Here's how the part is built. I have some questions about the finished solid (model axes, mm). A direction names the side the tool comes from. Round coordinates to 2 decimals unless told otherwise and drop trailing zeros. Write each loop counter-clockwise with the first axis right and the second up, starting at its lowest first coordinate (ties: lowest second). Pieces come first, ordered by that corner, then holes. Notation, with made-up numbers: (-22.5, 58) -> (0.5, 58) arc R32 ccw to (0.5, 92) -> close; hole circle Ø11 at (79.5, -2.5). An arc over 180 degrees is marked (long way). Answer as CSV lines item,"result".
Autodesk Inventor part; units mm, degrees
ref_plane "dp1_XY" through (7.9502, 4.7307, 0) normal (0, 0, 1) x (1, 0, 0)
ref_plane "dp1_YZ" through (7.9502, 4.7307, 0) normal (1, 0, 0) x (0, 1, 0)
ref_plane "dp1_ZX" through (7.9502, 4.7307, 0) normal (0, 1, 0) x (0, 0, 1)
sketch "Sketch_2" plane through (0, 0, 0) normal (0, 0, 1) x (1, 0, 0)
  line L0 (7.9502, 0) -> (0, 0)
  line L1 (0, 0) -> (0, 4.1326)
  line L2 (0, 4.1326) -> (0.6299, 4.7625)
  line L3 (0.6299, 4.7625) -> (3.9106, 4.7625)
  line L4 (3.9106, 4.7625) -> (4.5411, 4.1336)
  arc A0 (4.5411, 4.1336) -> (5.0165, 3.937) centre (5.0165, 4.6101) ccw
  line L5 (5.0165, 3.937) -> (6.0071, 3.937)
  arc A1 (6.0071, 3.937) -> (6.6802, 4.6101) centre (6.0071, 4.6101) ccw
  line L6 (6.6802, 4.6101) -> (6.6802, 4.7307)
  line L7 (6.6802, 4.7307) -> (7.9502, 4.7307)
  line L8 (7.9502, 4.7307) -> (7.9502, 0)
  line L9 (7.9502, 0) -> (0, 0)
revolve "Revolution1" add sketch "Sketch_2" angle 360 about axis through (7.9502, 0, 0) along (1, 0, 0)
thread "Thread1"
sketch "Sketch_3" plane through (0, 0, 0) normal (0, 0, 1) x (1, 0, 0)
  line L0 (15.9004, 0) -> (7.9502, 0)
  line L1 (7.9502, 0) -> (7.9502, 6.1468)
  line L2 (7.9502, 6.1468) -> (11.1252, 6.1468)
  line L3 (11.1252, 6.1468) -> (11.1252, 5.1626)
  line L4 (11.1252, 5.1626) -> (11.6332, 5.1626)
  line L5 (11.6332, 5.1626) -> (12.1412, 5.6706)
  line L6 (12.1412, 5.6706) -> (15.3924, 5.6706)
  line L7 (15.3924, 5.6706) -> (15.9004, 5.1626)
  line L8 (15.9004, 5.1626) -> (15.9004, 0)
  line L9 (15.9004, 0) -> (7.9502, 0)
revolve "Revolution2" add sketch "Sketch_3" angle 360 about axis through (15.9004, 0, 0) along (1, 0, 0)
sketch "Sketch_4" plane through (0, 0, 0) normal (0, 0, 1) x (1, 0, 0)
  line L0 (17.4752, 0) -> (15.9004, 0)
  line L1 (15.9004, 0) -> (15.9004, 4.4069)
  line L2 (15.9004, 4.4069) -> (17.4752, 4.4069)
  line L3 (17.4752, 4.4069) -> (17.4752, 0)
  line L4 (17.4752, 0) -> (15.9004, 0)
revolve "Revolution3" add sketch "Sketch_4" angle 360 about axis through (17.4752, 0, 0) along (1, 0, 0)
sketch "Sketch4" plane through (0, 0, 0) normal (-1, 0, 0) x (0, 0, 1)
  point P0 (0, 0)
hole "Hole1" at (0, 0, 0) direction (1, 0, 0) diameter 4.8133 depth 17.4752 countersink diameter 5.8293 countersink angle 90
sketch "Sketch_47" plane through (0, 0, 0) normal (0, 0, 1) x (1, 0, 0)
  line L0 (11.6332, 0) -> (11.1252, 0)
  line L1 (11.1252, 5.6603) -> (11.1252, 4.9085)
  line L2 (11.1252, 4.9085) -> (11.6332, 4.9085)
  line L3 (11.6332, 4.9085) -> (11.6332, 5.1626)
  line L4 (11.6332, 5.1626) -> (11.3792, 5.1626)
  line L5 (11.3792, 5.1626) -> (11.2368, 5.305)
  arc A0 (11.2368, 5.4846) -> (11.2368, 5.305) centre (11.3266, 5.3948) ccw
  line L6 (11.2368, 5.4846) -> (11.8149, 6.0626)
  line L7 (11.8149, 6.0626) -> (11.8149, 6.1468)
  line L8 (11.8149, 6.1468) -> (11.6117, 6.1468)
  line L9 (11.6117, 6.1468) -> (11.1252, 5.6603)
revolve "Revolution4" add sketch "Sketch_47" angle 360 about axis through (11.6332, 0, 0) along (1, 0, 0)
ref_plane "dp1_XY" through (7.9502, 4.7307, 0) normal (0, 0, 1) x (1, 0, 0)
ref_plane "dp1_YZ" through (7.9502, 4.7307, 0) normal (1, 0, 0) x (0, 1, 0)
ref_plane "dp1_ZX" through (7.9502, 4.7307, 0) normal (0, 1, 0) x (0, 0, 1)
ref_plane "dp2_XY" through (7.9502, -4.7307, 0) normal (0, 0, 1) x (1, 0, 0)
ref_plane "dp2_YZ" through (7.9502, -4.7307, 0) normal (1, 0, 0) x (0, 1, 0)
ref_plane "dp2_ZX" through (7.9502, -4.7307, 0) normal (0, 1, 0) x (0, 0, 1)
ref_plane "hh_XY" through (0, 4.7625, 0) normal (0, 0, 1) x (1, 0, 0)
ref_plane "hh_YZ" through (0, 4.7625, 0) normal (1, 0, 0) x (0, 1, 0)
ref_plane "hh_ZX" through (0, 4.7625, 0) normal (0, 1, 0) x (0, 0, 1)
ref_plane "rod_guide_XY" through (0, 0, 0) normal (1, 0, 0) x (0, 0, -1)
ref_plane "rod_guide_YZ" through (0, 0, 0) normal (0, 0, -1) x (0, 1, 0)
ref_plane "rod_guide_ZX" through (0, 0, 0) normal (0, 1, 0) x (1, 0, 0)
ref_plane "s1_XY" through (6.6802, 0, 0) normal (0, 0, 1) x (1, 0, 0)
ref_plane "s1_YZ" through (6.6802, 0, 0) normal (1, 0, 0) x (0, 1, 0)
ref_plane "s1_ZX" through (6.6802, 0, 0) normal (0, 1, 0) x (0, 0, 1)
ref_plane "s2_XY" through (7.9502, 0, 0) normal (0, 0, 1) x (1, 0, 0)
ref_plane "s2_YZ" through (7.9502, 0, 0) normal (1, 0, 0) x (0, 1, 0)
ref_plane "s2_ZX" through (7.9502, 0, 0) normal (0, 1, 0) x (0, 0, 1)
ref_plane "t1_XY" through (7.9502, 0, 0) normal (1, 0, 0) x (0, 0, -1)
ref_plane "t1_YZ" through (7.9502, 0, 0) normal (0, 0, -1) x (0, 1, 0)
ref_plane "t1_ZX" through (7.9502, 0, 0) normal (0, 1, 0) x (1, 0, 0)
ref_plane "t111_XY" through (7.9502, 0, 0) normal (1, 0, 0) x (0, 0, -1)
ref_plane "t111_YZ" through (7.9502, 0, 0) normal (0, 0, -1) x (0, 1, 0)
ref_plane "t111_ZX" through (7.9502, 0, 0) normal (0, 1, 0) x (1, 0, 0)
ref_plane "to_foot_bracket_XY" through (7.9502, 0, 0) normal (1, 0, 0) x (0, 0, -1)
ref_plane "to_foot_bracket_YZ" through (7.9502, 0, 0) normal (0, 0, -1) x (0, 1, 0)
ref_plane "to_foot_bracket_ZX" through (7.9502, 0, 0) normal (0, 1, 0) x (1, 0, 0)
ref_plane "to_nut_XY" through (6.6802, 0, 0) normal (1, 0, 0) x (0, 0, -1)
ref_plane "to_nut_YZ" through (6.6802, 0, 0) normal (0, 0, -1) x (0, 1, 0)
ref_plane "to_nut_ZX" through (6.6802, 0, 0) normal (0, 1, 0) x (1, 0, 0)
ref_plane "to_rod_XY" through (0, 0, 0) normal (1, 0, 0) x (0, 0, -1)
ref_plane "to_rod_YZ" through (0, 0, 0) normal (0, 0, -1) x (0, 1, 0)
ref_plane "to_rod_ZX" through (0, 0, 0) normal (0, 1, 0) x (1, 0, 0)
ref_plane "to_screw_XY" through (5.588, 0, 0) normal (0, 1, 0) x (1, 0, 0)
ref_plane "to_screw_YZ" through (5.588, 0, 0) normal (1, 0, 0) x (0, 0, -1)
ref_plane "to_screw_ZX" through (5.588, 0, 0) normal (0, 0, -1) x (0, 1, 0)
ref_plane "to_trunnion_brackets_XY" through (7.9248, 0, 0) normal (0, 1, 0) x (1, 0, 0)
ref_plane "to_trunnion_brackets_YZ" through (7.9248, 0, 0) normal (1, 0, 0) x (0, 0, -1)
ref_plane "to_trunnion_brackets_ZX" through (7.9248, 0, 0) normal (0, 0, -1) x (0, 1, 0)
ref_plane "to_trunnion_brackets1_XY" through (7.9248, 9.525, 0) normal (0, 1, 0) x (1, 0, 0)
ref_plane "to_trunnion_brackets1_YZ" through (7.9248, 9.525, 0) normal (1, 0, 0) x (0, 0, -1)
ref_plane "to_trunnion_brackets1_ZX" through (7.9248, 9.525, 0) normal (0, 0, -1) x (0, 1, 0)
ref_plane "to_trunnion_brackets2_XY" through (7.9248, -9.525, 0) normal (0, 1, 0) x (1, 0, 0)
ref_plane "to_trunnion_brackets2_YZ" through (7.9248, -9.525, 0) normal (1, 0, 0) x (0, 0, -1)
ref_plane "to_trunnion_brackets2_ZX" through (7.9248, -9.525, 0) normal (0, 0, -1) x (0, 1, 0)
ref_plane "to_tube_XY" through (11.6332, 0, 0) normal (1, 0, 0) x (0, 0, -1)
ref_plane "to_tube_YZ" through (11.6332, 0, 0) normal (0, 0, -1) x (0, 1, 0)
ref_plane "to_tube_ZX" through (11.6332, 0, 0) normal (0, 1, 0) x (1, 0, 0)
properties part number "01000-0_rod_guide"
1. Suppose I cut it at A-A on x = 7.5. Please give me the cut outline in (y, z).
Numbers:
outline,"circle Ø9.46 at (0, 0); hole circle Ø4.81 at (0, 0)"
2. If we mould it in two halves opening along Z, with no side actions, what happens to faces 4 (the face through (0, -3, -1)), 5 (the face through (5.519, -0.853, -3.843)), 6 (the face through (9.11, 1.464, -1.91))? For each: released by +Z, released by -Z, zero draft, split by the parting line, or undercut.
Numbers:
face 4,"zero draft"
face 5,"split by the parting line"
face 6,"undercut"
3. On a 3-axis mill with a long thin cutter (end or side, diameter ignored), from which of +Z, -Z, +X, -X, +Y, -Y can I reach the whole of each face in a straight line? I mean faces 1 (the face through (2.29, -3.78, -2.9)), 2 (the face through (16.7, -0.96, -4.3)), 3 (the face through (9.56, 5.86, 1.85)). Say none if no direction works.
Numbers:
face 1,"-X"
face 2,"+X"
face 3,"+X, -X"
4. For pin 1 Ø3 at (y, z) = (-2, 0) entering from +X; pin 2 Ø1.5 at (x, z) = (13, 3) entering from +Y; pin 3 Ø6 at (x, y) = (10, -3.5) entering from -Z; pin 4 Ø3 at (x, z) = (6, -2.5) entering from -Y, each with a flat end and sliding along its axis, tell me the tip position at first contact or that it passes through.
Numbers:
pin 1,"stops at x = 17.48"
pin 2,"stops at y = 5.21"
pin 3,"stops at z = -6.13"
pin 4,"stops at y = -4.59"
5. If I drill on line 1 (Z direction, x = 13.75, y = 0); line 2 (Y direction, x = 11.25, z = 3.75); line 3 (Z direction, x = 10.5, y = 0), over which ranges is the centre line in solid material (lowest first)?
Numbers:
line 1,"z = -5.67 to -2.41, 2.41 to 5.67"
line 2,"y = -4.41 to -4.02, -3.73 to 3.73, 4.02 to 4.41"
line 3,"z = -6.15 to -2.41, 2.41 to 6.15"
